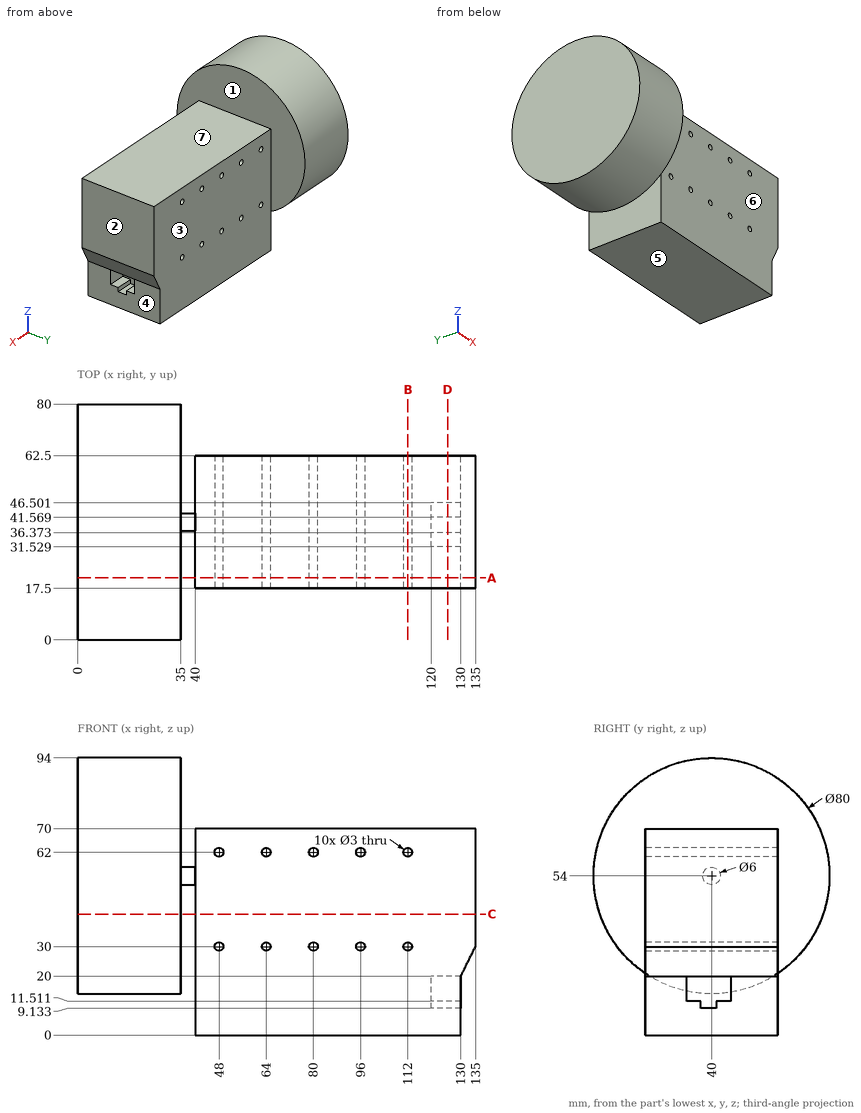
For this review, use the dimensioned drawing (mm, ordinates from the lowest corner) and the shaded views. A direction names the side the tool comes from. Give positions to 0.01 mm unless a question says otherwise; leave off trailing zeros. Write each loop counter-clockwise with the first axis right and the second up, starting at its lowest first coordinate (ties: lowest second). Pieces come first, ordered by that corner, then holes.
(1) The part is to be moulded in two halves that separate along X. For the marked faces 1, 2 and 3, say which applies: released by +X, released by -X, zero draft, split by the parting line, or undercut.
(2) Consider section B-B, the plane x = 112. Give the boundary of the cut face in (y, z).
(3) Consider section D-D, the plane x = 125.5. Give the boundary of the cut face in (y, z), and give its area (3 significant figures).
(4) Consider section A-A, the plane y = 21. Give the number of separate pieces and of enclosed holes in the cut face, and give its area (3 significant figures).
(5) Consider section C-C, the plane z = 41. Give the boundary of the cut face in (x, y).
(6) For P1, Ø2.5, axis at x = 48, z = 62, coming from the +Y side; P2, Ø21, axis at x = 107.5, z = 48, coming from the -Y side; P3, Ø3, axis at x = 33, y = 24.5, coming from the +Z side; P4, Ø4, axis at x = 127, z = 14, coming from the +Y side, all flat-tipped, find the tip position at first contact; note any pin that passes through.
(7) To check wall thickness, follow L1, parallel to Z at x = 48, y = 53; L2, parallel to Y at x = 112.5, z = 48.5; L3, parallel to X at y = 27, z = 77. State the ranges of each line that lie inside material, in increasing order.
(8) Tool access review of the marked faces 4, 5, 6 and 7: name each direction out of +Z, -Z, +X, -X, +Y, -Y from which nothing blocks a thin tool from reaching the whole face with its end or side.
Returned:
1. face 1: undercut
1. face 2: released by +X
1. face 3: zero draft
2. outline: (17.5, 0) - (62.5, 0) - (62.5, 28.5) - (17.5, 28.5) - close; (17.5, 31.5) - (62.5, 31.5) - (62.5, 60.5) - (17.5, 60.5) - close; (17.5, 63.5) - (62.5, 63.5) - (62.5, 70) - (17.5, 70) - close
3. outline: (17.5, 0) - (62.5, 0) - (62.5, 70) - (17.5, 70) - close; hole (31.53, 11.51) - (36.37, 11.51) - (36.37, 9.13) - (41.57, 9.13) - (41.57, 11.51) - (46.5, 11.51) - (46.5, 20) - (31.53, 20) - close
3. area: 3,010 mm2
4. separate pieces: 2
4. enclosed holes: 10
4. area: 8,920 mm2
5. outline: (0, 2.17) - (35, 2.17) - (35, 77.83) - (0, 77.83) - close; (40, 17.5) - (135, 17.5) - (135, 62.5) - (40, 62.5) - close
6. P1: passes through
6. P2: stops at y = 17.5
6. P3: stops at z = 91.47
6. P4: stops at y = 62.5
7. L1: z = 0 to 28.5, 31.5 to 60.5, 63.5 to 70
7. L2: y = 17.5 to 62.5
7. L3: x = 0 to 35
8. face 4: -Z, +X, +Y, -Y
8. face 5: -Z, +X, -X, +Y, -Y
8. face 6: +Z, -Z, +X, -Y
8. face 7: +Z, +X, +Y, -Y
